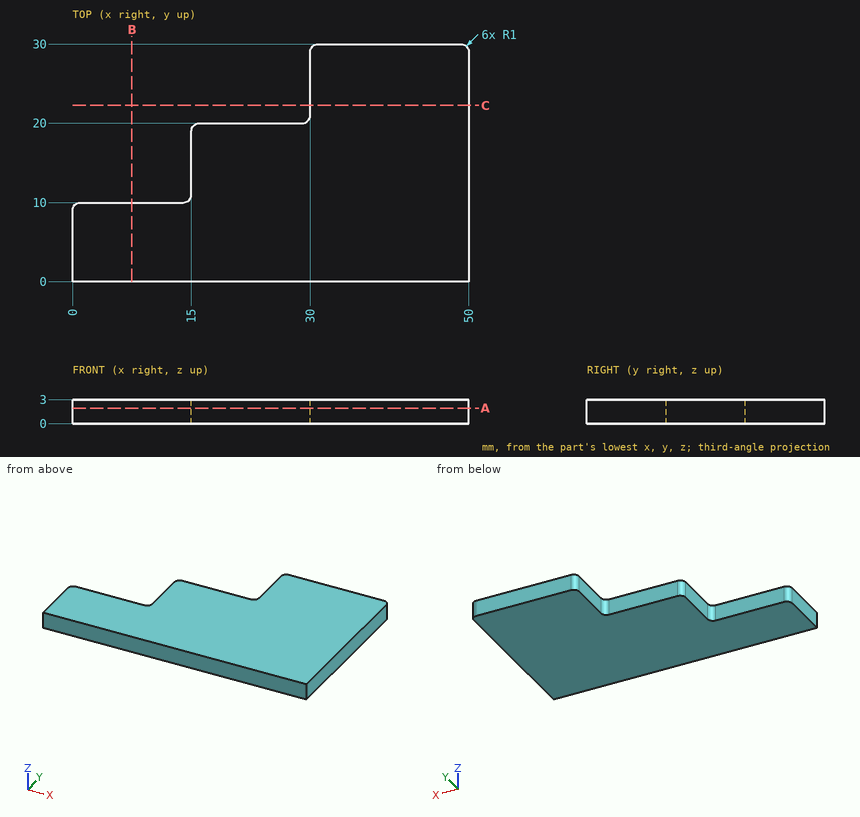
Geometry: see drawing. Coordinates: mm, zero at the bounding-box minimum. Give positions to 0.01 mm unless a question says otherwise; leave off trailing zeros. Order: outer loops, then holes, each group sorted by start corner. A loop starts at its lowest first (then second) coordinate and runs counter-clockwise, first axis right, second up.
Q1. Section C-C on y = 22.25. Output: boundary loops of the cut face in (x, z), and give its area (3 significant figures).
Checked values:
outline: (30, 0) - (50, 0) - (50, 3) - (30, 3) - close
area: 60.0 mm2
Q2. Ray query, probe 1 along Y at (x, z) = (18, 1.1); probe 2 along X at (y, z) = (12.75, 2); probe 3 along X at (y, z) = (24, 0.5). Return the intervals inside material, ascending.
Checked values:
probe 1: y = 0 to 20
probe 2: x = 15 to 50
probe 3: x = 30 to 50
Q3. Section A-A on z = 1.95. Output: boundary loops of the cut face in (x, y), and give its area (3 significant figures).
Checked values:
outline: (0, 0) - (50, 0) - (50, 29) arc R1 ccw to (49, 30) - (31, 30) arc R1 ccw to (30, 29) - (30, 21) arc R1 cw to (29, 20) - (16, 20) arc R1 ccw to (15, 19) - (15, 11) arc R1 cw to (14, 10) - (1, 10) arc R1 ccw to (0, 9) - close
area: 1,050 mm2
Q4. Section B-B on x = 7.5. Output: boundary loops of the cut face in (y, z).
Checked values:
outline: (0, 0) - (10, 0) - (10, 3) - (0, 3) - close
Q5. Contact query for flat-ended pins moving along their axis: pin 1 Ø1 at (x, z) = (37, 1) entering from -Y; pin 2 Ø1.5 at (y, z) = (26.5, 0.5) entering from -X; pin 3 Ø1 at (y, z) = (11.5, 0.5) entering from -X; pin 4 Ø0.9 at (x, z) = (23, 1.5) entering from +Y. Output: stop coordinate, or through.
Checked values:
pin 1: stops at y = 0
pin 2: stops at x = 30
pin 3: stops at x = 15
pin 4: stops at y = 20
